Job drawing, mm, ordinate dimensions from the low corner. One solid piece. Give positions to 0.01 mm unless a question says otherwise; leave off trailing zeros. Loops run counter-clockwise (first coordinate to the right, second up) from the corner with the lowest first, then second, coordinate; pieces in that order, holes last. Notation, with made-up numbers: (39, 66) -> (66, 66) arc R10 ccw to (66, 83) -> close; hole circle Ø10 at (82, 18.5). An arc over 180 degrees is marked (long way). Use one line per item in the form item = value.
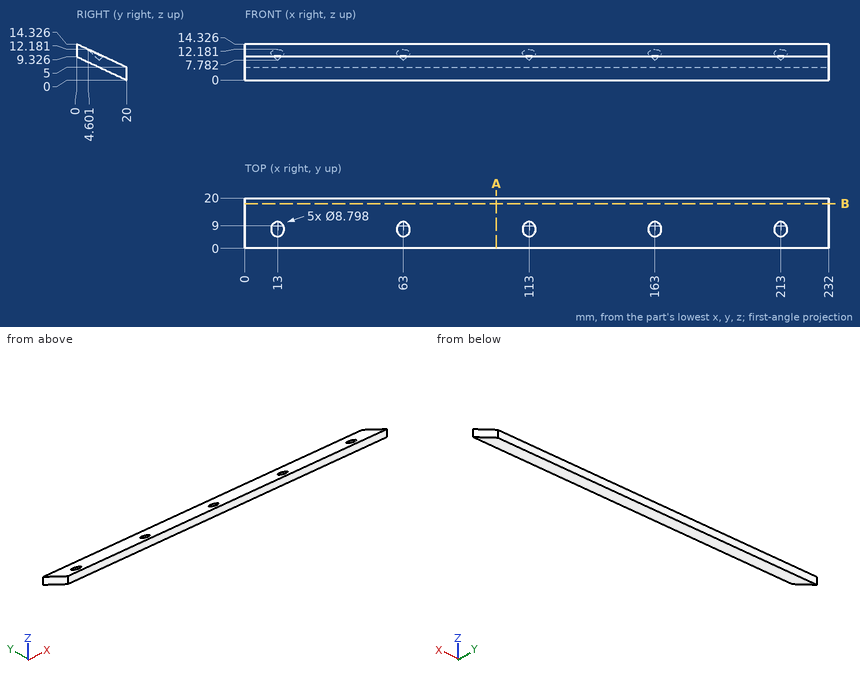
1. Drop flat-ended pins along their axis: P1, Ø1, axis at x = 131.5, y = 7, coming from the +Z side (1 decimal); P2, Ø1.5, axis at x = 113.5, y = 3, coming from the +Z side; P3, Ø1, axis at x = 116, z = 3, coming from the -Y side (1 decimal). Give the stop position or say it passes through.
Result sheet:
P1 = 11.3
P2 = 13.28
P3 = 12.5
2. Cut at B-B, the plane y = 17.75. Write the cut outline in (x, z), then the cut area to 3 significant figures.
Result sheet:
outline = (0, 1.05) -> (232, 1.05) -> (232, 6.05) -> (0, 6.05) -> close
area = 1,160 mm^2
3. Drill centre lines: line 1 (Y direction, x = 84, z = 13) (1 decimal); line 2 (Z direction, x = 133, y = 16.25); line 3 (Y direction, x = 32, z = 7) (1 decimal). Where is each one in solid material? Low to high.
Result sheet:
line_1 = 0 to 2.8
line_2 = 1.75 to 6.75
line_3 = 5 to 15.7
4. Cut at A-A, the plane x = 100. Write the cut outline in (y, z), then the cut area to 3 significant figures.
Result sheet:
outline = (0, 9.33) -> (20, 0) -> (20, 5) -> (0, 14.33) -> close
area = 100 mm^2
